Geometry: final body of the model. Coordinates: model frame, mm. A direction names the side the tool comes from. Coordinates: 2 decimals unless noted, no trailing zeros. Loops run counter-clockwise (first coordinate to the right, second up) from the corner with the lowest first, then second, coordinate; pieces in that order, holes last. Notation, with made-up numbers: M 46,60.5 L 102,60.5 A18 cw 102,77.5 Z; hole C -8.75,10 d10. An arc over 180 degrees is marked long. Write each question's results on one line, items separated by ' | '. Start each with the question number.
from build123d import *

# Parameters (mm, degrees)
SKETCH1_R           = 9.525
BOSS_EXTRUDE1_DEPTH = 6.35
SKETCH2_W           = 6.35
SKETCH2_H           = 11.43
BOSS_EXTRUDE2_DEPTH = 25.4
CUT_EXTRUDE1_DEPTH  = 25.4
SKETCH4_R           = 2.4892
CUT_EXTRUDE2_DEPTH  = 12.7
FILLET1_R           = 2.54


with BuildPart() as part:
    # Sketch1 → Boss-Extrude1 (new body)
    with BuildSketch(Plane.XY):
        with BuildLine():
            Line((19.05, 0), (19.05, 24.13))
            ThreePointArc((19.05, 24.13), (0, 43.18), (-19.05, 24.13))
            Line((-19.05, 24.13), (-19.05, 0))
            Line((-19.05, 0), (19.05, 0))
        make_face()
        with Locations((0, 24.13)):
            Circle(SKETCH1_R, mode=Mode.SUBTRACT)
    extrude(amount=BOSS_EXTRUDE1_DEPTH)

    # Sketch2 → Boss-Extrude2 (add)
    with BuildSketch(Plane.XY.offset(6.35)):
        with Locations((0, 5.715)):
            Rectangle(SKETCH2_W, SKETCH2_H)
    extrude(amount=BOSS_EXTRUDE2_DEPTH)

    # Sketch3 → Cut-Extrude1 (cut)
    with BuildSketch(Plane(origin=(3.175, 0, 0), x_dir=(0, 0, -1), z_dir=(1, 0, 0))):
        Polygon((-31.75, 5.715), (-19.05, 11.43), (-31.75, 11.43), align=None)
    extrude(amount=-CUT_EXTRUDE1_DEPTH, mode=Mode.SUBTRACT)

    # Sketch4 → Cut-Extrude2 (cut)
    with BuildSketch(Plane.XZ):
        with Locations(Location((-9.525, 3.175, 0), (0, 0, 270))):
            Circle(SKETCH4_R)
        with Locations(Location((9.525, 3.175, 0), (0, 0, 270))):
            Circle(SKETCH4_R)
        with Locations(Location((0, 22.86, 0), (0, 0, 270))):
            Circle(SKETCH4_R)
    extrude(amount=-CUT_EXTRUDE2_DEPTH, mode=Mode.SUBTRACT)

    # Fillet1
    fillet1_edges = [part.edges().sort_by_distance(p)[0] for p in [
        (0, 11.43, 19.05),
        (3.175, 5.715, 6.35),
        (0, 11.43, 6.35),
        (-3.175, 5.715, 6.35),
    ]]
    fillet(fillet1_edges, radius=FILLET1_R)


solid = part.part
Item 1: Ray query, L1, parallel to X at y = 4.5, z = 22.86 (3 decimals); L2, parallel to Z at x = -6, y = 14. Return the intervals inside material, ascending. Write a range as [from, to].
Item 2: Pull-direction query (X, two-part tool) for faces 6 (the flat face through (0, 3, 31.75)), 7 (the cylindrical face through (-3.939, 5.531, 7.074)), 8 (the cylindrical face through (-11.04, 6.26, 5.15)); classes: released by +X, released by -X, zero draft, split by the parting line, or undercut.
Item 3: Section C-C, the plane x = 1. Count the separate pieces of the cut face and the enclosed holes in it, plus the area to 3 significant figures.
Item 4: Section B-B, the plane z = 22.86. Return loops of the section in (x, y) (1 decimal), plus the area to 3 significant figures.
Item 5: Set-up query: faces 1 (the cylindrical face through (11.993, 6.261, 3.499)), 2 (the flat face through (-3.175, 6, 20)), 3 (the flat face through (8, 17, 6.35)), 4 (the cylindrical face through (0.419, 43.175, 3.131)), 5 (the flat face through (0, 11.43, 14)). Return all of +Z, -Z, +X, -X, +Y, -Y with unobstructed straight access to the full face (end or side cutting, diameter ignored); none if empty.
Item 6: Contact query for flat-ended pins moving along their axis: P1, Ø5, axis at x = -1.5, z = 14.5, coming from the +Y side; P2, Ø1.5, axis at x = -5, y = 33, coming from the +Z side; P3, Ø9, axis at y = 6, z = 18, coming from the +X side (3 decimals); P4, Ø10, axis at y = 21, z = 21.5, coming from the +X side. Output: stop coordinate, or through.
Item 7: Section D-D, the plane x = -5. Return loops of the section in (y, z) (3 decimals).
Item 8: Section A-A, the plane y = 19.5. Return loops of the section in (x, z).
Solutions:
1) L1: x = [-3.175, -2.489], [2.489, 3.175] | L2: z = [0, 6.35]
2) face 6: zero draft | face 7: released by -X | face 8: undercut
3) separate pieces: 3 | enclosed holes: 0 | area: 365 mm²
4) outline: M -3.2,0 L -2.5,0 L -2.5,9.7 L -3.2,9.7 Z; M 2.5,0 L 3.2,0 L 3.2,9.7 L 2.5,9.7 Z | area: 13.3 mm²
5) face 1: -Y | face 2: +Z, -X, +Y, -Y | face 3: +Z, +Y | face 4: +Z, -Z, +Y | face 5: +Z, +X, -X, +Y
6) P1: stops at y = 11.43 | P2: stops at z = 6.35 | P3: stops at x = 3.175 | P4: passes through
7) outline: M 0,0 L 16.023,0 L 16.023,6.35 L 13.97,6.35 A2.54 cw 13.255,6.453 L 0,6.453 Z; M 32.237,0 L 42.512,0 L 42.512,6.35 L 32.237,6.35 Z
8) outline: M -19.05,0 L -8.32,0 L -8.32,6.35 L -19.05,6.35 Z; M 8.32,0 L 19.05,0 L 19.05,6.35 L 8.32,6.35 Z
